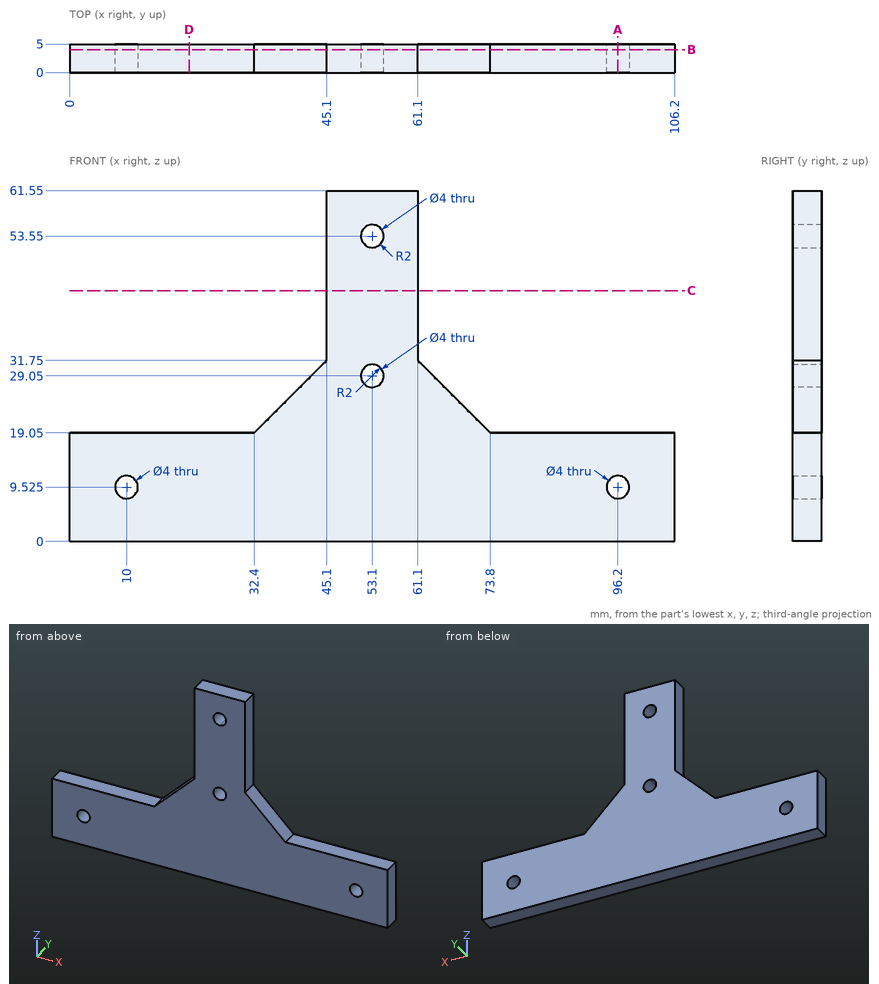
Answer from the drawing. Dimensions are ordinates in mm from the lowest x, y and z of the part. Coordinates: 2 decimals unless noted, no trailing zeros. Order: outer loops, then holes, each group sorted by start corner. A loop starts at its lowest first (then second) coordinate and runs counter-clockwise, first axis right, second up. Notation, with made-up numbers: (19, 82) -> (51, 82) arc R25 ccw to (51, 118) -> close; hole circle Ø11 at (17.5, 18.25). An arc over 180 degrees is marked (long way). Answer as a JSON object with one key per item and string values.
1) A cutting plane is placed at B-B, the plane y = 4. Determine the outline of the cut face in (x, z) (3 decimals), plus the area to 3 significant figures.
Model answer:
{"outline": "(0, 0) -> (106.2, 0) -> (106.2, 19.05) -> (73.8, 19.05) -> (61.1, 31.75) -> (61.1, 61.55) -> (45.1, 61.55) -> (45.1, 31.75) -> (32.4, 19.05) -> (0, 19.05) -> close; hole circle Ø4 at (10, 9.525); hole circle Ø4 at (53.1, 29.05); hole circle Ø4 at (53.1, 53.55); hole circle Ø4 at (96.2, 9.525)", "area": "2,810 mm²"}
2) A cutting plane is placed at D-D, the plane x = 21. Determine the outline of the cut face in (y, z), plus the area to 4 significant figures.
Model answer:
{"outline": "(0, 0) -> (5, 0) -> (5, 19.05) -> (0, 19.05) -> close", "area": "95.25 mm²"}
3) A cutting plane is placed at C-C, the plane z = 44. Determine the outline of the cut face in (x, y), plus the area to 3 significant figures.
Model answer:
{"outline": "(45.1, 0) -> (61.1, 0) -> (61.1, 5) -> (45.1, 5) -> close", "area": "80.0 mm²"}
4) Each of these flat-tipped pins is pushed along its axis until it touches: pin 1 (4 mm diameter, centred on x = 43, z = 32, fed in from +Y); pin 2 (1.5 mm diameter, centred on y = 2, z = 41, fed in from +X); pin 3 (2 mm diameter, centred on x = 90, y = 3, fed in from +Z); pin 4 (1.5 mm diameter, centred on y = 3.5, z = 43.5, fed in from -X). Where does it stop, or does it pass through?
Model answer:
{"pin 1": "stops at y = 5", "pin 2": "stops at x = 61.1", "pin 3": "stops at z = 19.05", "pin 4": "stops at x = 45.1"}
5) Consider line 1 along Z through (x, y) = (53.1, 2.8); line 2 along X through (y, z) = (3.85, 53.55); line 3 along X through (y, z) = (1, 11). Determine where each line is inside the solid, lowest interval first. Write a range as from..to.
Model answer:
{"line 1": "z = 0..27.05, 31.05..51.55, 55.55..61.55", "line 2": "x = 45.1..51.1, 55.1..61.1", "line 3": "x = 0..8.65, 11.35..94.85, 97.55..106.2"}
6) A cutting plane is placed at A-A, the plane x = 96.2. Determine the outline of the cut face in (y, z) (3 decimals).
Model answer:
{"outline": "(0, 0) -> (5, 0) -> (5, 7.525) -> (0, 7.525) -> close; (0, 11.525) -> (5, 11.525) -> (5, 19.05) -> (0, 19.05) -> close"}
